Geometry check sheet. Reference: the model listing, model coordinates, mm. Face numbers are marked on the shaded views. A direction names the side the tool comes from. Give positions to 0.01 mm unless a question says otherwise; leave off trailing zeros. Loops run counter-clockwise (first coordinate to the right, second up) from the corner with the lowest first, then second, coordinate; pieces in that order, holes last. Notation, with made-up numbers: (23, 50) -> (75, 50) arc R17 cw to (75, 62) -> close; hole circle Ø9 at (64.5, 81). An arc over 180 degrees is marked (long way). Write each question's results on one line, items separated by ' | '. Start each with the question number.
1) Sectioned sample at B-B on y = 20.5. Record the cut outline in (x, z), then the cut area to 3 significant figures.
2) Set-up check for the marked faces 4 and 5: record each of +Z, -Z, +X, -X, +Y, -Y from which the full face is reachable in a straight line by a thin tool's end or side.
3) Sectioned sample at A-A on x = 41.5. Record the cut outline in (y, z) (3 decimals), then the cut area to 3 significant figures.
4) Scan lines: line 1 (Z direction, x = 52.5, y = 94.4) (3 decimals); line 2 (X direction, y = 93.5, z = -43.5) (3 decimals); line 3 (X direction, y = 93.05, z = 43.5) (3 decimals). Record each from-to range of solid material in increasing order. Write a range as from..to.
5) Sectioned sample at C-C on z = 21.5. Record the cut outline in (x, y) (3 decimals), then the cut area to 3 significant figures.
6) Depth check by flat-ended pin: pin 1 (5.5 mm diameter, centred on x = -1, y = 91.5, fed in from +Z); pin 2 (1.6 mm diameter, centred on x = 10.5, z = 42.5, fed in from +Y); pin 3 (6 mm diameter, centred on x = 53.5, z = -43, fed in from +Y); pin 4 (2 mm diameter, centred on y = 54.5, z = 29, fed in from -X). Enter the tip coordinate at first touch or a pass-through.
7) Draft check along Z on the marked faces 1, 2 and 3. Enter one of: pulls with the +Z half, pulls with the -Z half, needs draft (parallel to the pull), parting line crosses it, or undercut.
Autodesk Inventor part; units mm, degrees
ref_plane "YZ Plane" through (0, 0, 0) normal (1, 0, 0) x (0, 1, 0)
ref_plane "XZ Plane" through (0, 0, 0) normal (0, 1, 0) x (-1, 0, 0)
ref_plane "XY Plane" through (0, 0, 0) normal (0, 0, 1) x (1, 0, 0)
sketch "Sketch8" plane through (0, 0, 0) normal (0, 1, 0) x (-1, 0, 0)
  line L0 (-56.5, -47.5) -> (56.5, -47.5)
  line L1 (56.5, -47.5) -> (56.5, 47.5)
  line L2 (56.5, 47.5) -> (-56.5, 47.5)
  line L3 (-56.5, 47.5) -> (-56.5, -47.5)
  line L4 (-56.5, -47.5) -> (56.5, 47.5) construction
  line L5 (56.5, -47.5) -> (-56.5, 47.5) construction
  point P0 (0, 0)
  dimension "d26" = 113
  dimension "d27" = 95
extrude "Extrusion7" add sketch "Sketch8" along normal blind 95
sketch "Sketch9" plane through (0, 0, 0) normal (0, -1, 0) x (1, 0, 0)
  line L0 (-56.5, 47.5) -> (56.5, 47.5)
  line L1 (-56.5, -47.5) -> (56.5, -47.5)
  line L2 (56.5, -47.5) -> (56.5, 47.5)
  line L3 (56.5, 47.5) -> (-56.5, 47.5)
  line L4 (-56.5, 47.5) -> (-56.5, -47.5)
  line L5 (-56.5, -47.5) -> (56.5, 47.5) construction
  line L6 (56.5, -47.5) -> (-56.5, 47.5) construction
  line L7 (52.5, 43.5) -> (52.5, -43.5)
  line L8 (52.5, -43.5) -> (-56.5, -43.5)
  line L9 (-56.5, 43.5) -> (52.5, 43.5)
  line L10 (48.5, -39.5) -> (48.5, 39.5)
  line L11 (48.5, 39.5) -> (-56.5, 39.5)
  line L12 (-56.5, -39.5) -> (48.5, -39.5)
  line L13 (-54.3018, -43.5) -> (-54.3018, -45.6519)
  line L14 (-54.3018, 45.6519) -> (-54.3018, 43.5)
  line L15 (-49.9386, 39.5) -> (-49.9386, 41.9838)
  line L16 (-49.9386, -41.9838) -> (-49.9386, -39.5)
  point P0 (0, 0)
  dimension "d30" = 4
  dimension "d31" = 4
  dimension "d47" = 4
  dimension "d48" = 4
  dimension "d49" = 4
  dimension "d50" = 4
extrude "Extrusion8" cut sketch "Sketch9" against normal blind 115 contours L11 L10 L12 L4
extrude "Extrusion9" cut sketch "Sketch9" against normal blind 90 contours L9 L7 L8 L4 L12 L10 L11
sketch "Sketch10" plane through (0, 0, 0) normal (0, -1, 0) x (1, 0, 0)
  line L0 (56.5, -47.5) -> (-56.5, -47.5)
  line L1 (-56.5, -47.5) -> (-56.5, 47.5)
  line L2 (-56.5, 47.5) -> (56.5, 47.5)
  line L3 (56.5, 47.5) -> (56.5, -47.5)
  line L4 (56.5, -47.5) -> (-56.5, 47.5) construction
  line L5 (-56.5, -47.5) -> (56.5, 47.5) construction
  line L6 (-60.5, 51.5) -> (-60.5, -51.5)
  line L7 (-60.5, -51.5) -> (60.5, -51.5)
  line L8 (60.5, -51.5) -> (60.5, 51.5)
  line L9 (60.5, 51.5) -> (-60.5, 51.5)
  line L10 (-56.5, 47.5) -> (-60.5, 47.5)
  line L11 (-56.5, -47.5) -> (-60.5, -47.5)
  line L12 (-56.5, 47.5) -> (-56.5, 51.5)
  line L13 (-56.5, -47.5) -> (-56.5, -51.5)
  point P0 (0, 0)
  dimension "d36" = 4
extrude "Extrusion10" add sketch "Sketch10" against normal blind 5 contours L3 L2 L12 L9 L8 L7 L13 L0
sketch "Sketch11" plane through (0, 0, 0) normal (0, -1, 0) x (1, 0, 0)
  circle A0 centre (-75.5, 17.5) radius 135
  line L0 (52.5, 43.5) -> (52.5, -43.5)
  line L1 (60.5, -51.5) -> (60.5, 51.5)
  circle A1 centre (-75.5, 17.5) radius 110
  line L2 (10.168, -51.5) -> (60.5, -51.5)
  line L3 (60.5, -51.5) -> (60.5, 51.5)
  line L4 (60.5, 51.5) -> (29.1136, 51.5)
  line L5 (-56.5, 51.5) -> (60.5, 51.5)
  point P0 (0, 0)
  dimension "d39" = 270
  dimension "d41" = 136
  dimension "d42" = 220
extrude "Extrusion11" cut sketch "Sketch11" against normal blind 1.125 contours A0 L2 A1 L4 | A0 L4 L1 L2 picked at (50.9054, 12.6578)
sketch "Sketch12" plane through (0, 95, 0) normal (0, 1, 0) x (1, 0, 0)
  line L0 (-56.5, -43.5) -> (52.5, -43.5)
  circle A0 centre (52.5, -43.5) radius 2.625
  line L1 (52.5, 43.5) -> (52.5, -43.5)
  circle A1 centre (52.5, 43.5) radius 2.625
  line L2 (52.5, 43.5) -> (-56.5, 43.5)
  circle A2 centre (7.5, 43.5) radius 2.625
  circle A3 centre (9.525, -43.5) radius 2.625
  point P0 (0, 0)
  dimension "d51" = 5.25
  dimension "d52" = 5.25
  dimension "d53" = 5.25
  dimension "d54" = 5.25
  dimension "d57" = 45
extrude "Extrusion13" cut sketch "Sketch12" against normal blind 2.5
properties part number "Galvo Housing-01"
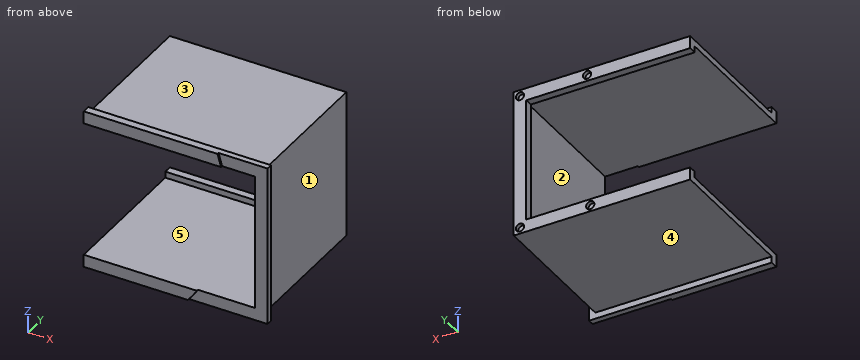
Result:
1) outline: (-56.5, -47.5) -> (56.5, -47.5) -> (56.5, 47.5) -> (-56.5, 47.5) -> (-56.5, 43.5) -> (52.5, 43.5) -> (52.5, -43.5) -> (-56.5, -43.5) -> close | area: 1,250 mm^2
2) face 4: -Z, +X, -X, +Y | face 5: -X, -Y
3) outline: (1.125, -51.5) -> (5, -51.5) -> (5, -47.5) -> (95, -47.5) -> (95, -39.5) -> (90, -39.5) -> (90, -43.5) -> (1.125, -43.5) -> close; (1.125, 43.5) -> (90, 43.5) -> (90, 39.5) -> (95, 39.5) -> (95, 47.5) -> (5, 47.5) -> (5, 51.5) -> (1.125, 51.5) -> close | area: 822 mm^2
4) line 1: -47.5..-46.125, -40.875..40.875, 46.125..47.5 | line 2: -56.5..4.875, 10.125..49.875, 55.125..56.5 | line 3: -56.5..6.9, 12.15..49.875, 55.125..56.5
5) outline: (48.5, 90) -> (52.5, 90) -> (52.5, 1.125) -> (60.5, 1.125) -> (60.5, 5) -> (56.5, 5) -> (56.5, 95) -> (48.5, 95) -> close | area: 411 mm^2
6) pin 1: z = 47.5 | pin 2: y = 92.5 | pin 3: y = 95 | pin 4: x = 52.5
7) face 1: needs draft | face 2: undercut | face 3: pulls with the +Z half
